The model under review builds one solid part; all positions refer to its coordinate system, in mm. Face numbers are marked on the shaded views. Give positions to 0.01 mm unless a question says otherwise; leave off trailing zeros. Loops run counter-clockwise (first coordinate to the right, second up) from the corner with the lowest first, then second, coordinate; pieces in that order, holes last. Notation, with made-up numbers: (7, -20) -> (19, -20) arc R21 ccw to (19, 0) -> close; hole circle Ø8 at (43.5, -13). An arc over 180 degrees is marked (long way). Write each question's results on one line, items separated by ' | '. Start each with the question number.
Q1. We need section C-C (z = 0). Write out the cut boundary in (x, y), plus the area to 3 significant figures.
Q2. We need section B-B (x = 0). Write out the cut boundary in (y, z).
Q3. Insertion check: pin 1 Ø1.5 at (x, z) = (22, -6.5) entering from -Y; pin 2 Ø1 at (y, z) = (26, 53.5) entering from -X; pin 3 Ø1 at (y, z) = (29, 77) entering from +X. Each pin has a flat end and moves straight along its axis. Give the tip position at first contact, or say it passes through.
Q4. We need section A-A (y = 24.5). Write out the cut boundary in (x, z), plus the area to 3 significant figures.
Q5. Wall thickness on L1, parallel to X at y = 8.75, z = 0; L2, parallel to Y at x = 65, z = 29.5; L3, parallel to Z at x = 1.5, y = 18: over which ranges is each line inside the solid? List them lowest first. Write a range as [from, to].
Q6. Mouldability with a two-part tool opening along X and no side actions: class the marked faces 1, 2, 3 and 4 as released by +X, released by -X, zero draft, split by the parting line, or undercut.
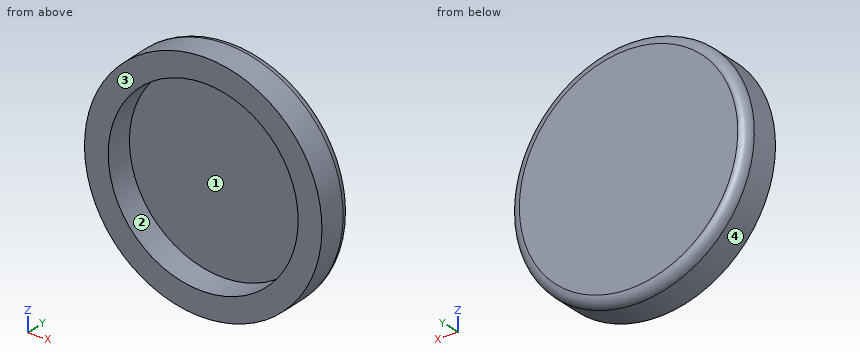
from build123d import *

# Parameters (mm, degrees)
CROQUIS1_R              = 125
SALIENTE_EXTRUIR1_DEPTH = 40
CROQUIS2_R              = 100
CORTAR_EXTRUIR1_DEPTH   = 30
REDONDEO1_R             = 10


with BuildPart() as part:
    # Croquis1 → Saliente-Extruir1 (new body)
    with BuildSketch(Plane(origin=(0, 0, 0), x_dir=(1, 0, 0), z_dir=(0, 1, 0))):
        with Locations(Location((0, 0, 0), (0, 0, 270))):
            Circle(CROQUIS1_R)
    extrude(amount=SALIENTE_EXTRUIR1_DEPTH)

    # Croquis2 → Cortar-Extruir1 (cut)
    with BuildSketch(Plane.XZ):
        with Locations(Location((0, 0, 0), (0, 0, 270))):
            Circle(CROQUIS2_R)
    extrude(amount=-CORTAR_EXTRUIR1_DEPTH, mode=Mode.SUBTRACT)

    # Redondeo1
    redondeo1_edges = [part.edges().sort_by_distance(p)[0] for p in [
        (0, 40, -125),
    ]]
    fillet(redondeo1_edges, radius=REDONDEO1_R)


solid = part.part
Output:
1) outline: (-125, 0) -> (-100, 0) -> (-100, 30) -> (100, 30) -> (100, 0) -> (125, 0) -> (125, 30) arc R10 ccw to (115, 40) -> (-115, 40) arc R10 ccw to (-125, 30) -> close | area: 3,960 mm2
2) outline: (0, -125) -> (30, -125) arc R10 ccw to (40, -115) -> (40, 115) arc R10 ccw to (30, 125) -> (0, 125) -> (0, 100) -> (30, 100) -> (30, -100) -> (0, -100) -> close
3) pin 1: y = 30 | pin 2: x = -113.21 | pin 3: x = 98.86
4) outline: circle Ø250 at (0, 0); hole circle Ø200 at (0, 0) | area: 17,700 mm2
5) L1: [-125, -100], [100, 125] | L2: [30, 40] | L3: [-124.99, -99.99], [99.99, 124.99]
6) face 1: undercut | face 2: undercut | face 3: zero draft | face 4: split by the parting line
